```python
from build123d import *

# Parameters (mm, degrees)
F0_W     = 101.6
F0_H     = 101.6
F1_DEPTH = 2743.2
F2_W     = 88.9
F2_H     = 88.9
F3_DEPTH = 2743.201
F4_R     = 5.08


with BuildPart() as f1:
    # F0 (on Top) → F1 (new body)
    with BuildSketch(Plane.XY):
        Rectangle(F0_W, F0_H)
    extrude(amount=F1_DEPTH)

    # F2 (on face) → F3 (cut, through all)
    with BuildSketch(Plane.XY.offset(2743.2)):
        Rectangle(F2_W, F2_H)
    extrude(amount=-F3_DEPTH, mode=Mode.SUBTRACT)

    # F4
    f4_edges = [f1.edges().sort_by_distance(p)[0] for p in [
        (50.8, -50.8, 1371.6),
        (50.8, 50.8, 1371.6),
        (-50.8, -50.8, 1371.6),
        (-50.8, 50.8, 1371.6),
    ]]
    fillet(f4_edges, radius=F4_R)


solid = f1.part
```
Check sheet for the modelled part. Datum: model origin and axes. Units: mm. A direction names the side the tool comes from. Round coordinates to 2 decimals unless told otherwise and drop trailing zeros. Write each loop counter-clockwise with the first axis right and the second up, starting at its lowest first coordinate (ties: lowest second). Pieces come first, ordered by that corner, then holes. Notation, with made-up numbers: (17, 9) -> (43, 9) arc R13 cw to (43, 29) -> close; hole circle Ø4 at (29, -6.75). An arc over 180 degrees is marked (long way). One line per question, with ' | ' between items. Start each with the question number.
1. Sectioned sample at C-C, the plane z = 2388. Record the cut outline in (x, y).
2. Set-up check for faces 4 (the face through (-44.45, -1, 1391)), 5 (the face through (-1, 50.8, 1352)): record each of +Z, -Z, +X, -X, +Y, -Y from which the full face is reachable in a straight line by a thin tool's end or side.
3. Release check for a two-part mould opening along Y. For faces 1 (the face through (50.8, -1, 1352)), 2 (the face through (-1, -50.8, 1352)), 3 (the face through (-1, 44.45, 1391)) record: +Y half, -Y half, draft (parallel to the pull), parting line (faces both ways), or undercut.
4. Sectioned sample at A-A, the plane x = -26.5. Record the cut outline in (y, z), then the cut area to 3 significant figures.
5. Scan line: line 1 along X through (y, z) = (-27, 830). Record every from-to range of solid material in increasing order. Write a range as from..to.
Taken from the geometry:
1) outline: (-50.8, -45.72) arc R5.08 ccw to (-45.72, -50.8) -> (45.72, -50.8) arc R5.08 ccw to (50.8, -45.72) -> (50.8, 45.72) arc R5.08 ccw to (45.72, 50.8) -> (-45.72, 50.8) arc R5.08 ccw to (-50.8, 45.72) -> close; hole (-44.45, -44.45) -> (44.45, -44.45) -> (44.45, 44.45) -> (-44.45, 44.45) -> close
2) face 4: +Z, -Z | face 5: +Z, -Z, +X, -X, +Y
3) face 1: draft | face 2: -Y half | face 3: undercut
4) outline: (-50.8, 0) -> (-44.45, 0) -> (-44.45, 2743.2) -> (-50.8, 2743.2) -> close; (44.45, 0) -> (50.8, 0) -> (50.8, 2743.2) -> (44.45, 2743.2) -> close | area: 34,800 mm^2
5) line 1: x = -50.8..-44.45, 44.45..50.8
